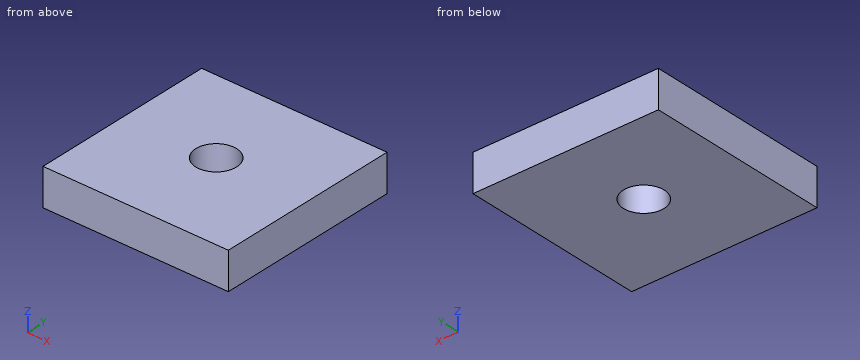
from build123d import *

# Parameters (mm, degrees)
F1_W     = 12.7
F1_H     = 12.7
F2_DEPTH = 2.54
F0_R     = 1.397
F3_DEPTH = 22.7076


with BuildPart() as f2:
    # F1 (on Top) → F2 (new body)
    with BuildSketch(Plane.XY):
        with Locations((0.047929, -0.151867)):
            Rectangle(F1_W, F1_H)
    extrude(amount=F2_DEPTH)

    # F0 (on Top) → F3 (cut)
    with BuildSketch(Plane.XY):
        Circle(F0_R)
    extrude(amount=F3_DEPTH, mode=Mode.SUBTRACT)


solid = f2.part
For this review, take the finished solid that the model builds, in its own axes (mm). Round coordinates to 2 decimals unless told otherwise and drop trailing zeros. Order: outer loops, then holes, each group sorted by start corner. A loop starts at its lowest first (then second) coordinate and runs counter-clockwise, first axis right, second up. Notation, with made-up numbers: M -33.5,-28.75 L -12.5,-28.75 A15 ccw -12.5,-11.75 Z; hole C 64.25,-18 d4. An arc over 180 degrees is marked long. Use a Markdown table: item, result. Add a question column.
Item 1: Add section C-C, the plane z = 2.2. Give the boundary of the cut face in (x, y).
Item 2: Add section B-B, the plane y = 0. Give the boundary of the cut face in (x, z), then the cut area to 3 significant figures.
Item 3: Insertion check: pin 1 (2 mm diameter, centred on x = 0, y = 0, fed in from -Z). The pin has a flat end and moves straight along its axis. Give the tip position at first contact, or say it passes through.
Item 4: Add section A-A, the plane x = 0. Give the boundary of the cut face in (y, z), then the cut area to 3 significant figures.
Item 5: To check wall thickness, follow line 1 along Y through (x, z) = (0, 0.6); line 2 along X through (y, z) = (0, 1.45); line 3 along Y through (x, z) = (1, 2.45). State the ranges of each line that lie inside material, in increasing order.
Geometry results:
| question | item | result |
|---|---|---|
| 1 | outline | M -6.3,-6.5 L 6.4,-6.5 L 6.4,6.2 L -6.3,6.2 Z; hole C 0,0 d2.79 |
| 2 | outline | M -6.3,0 L -1.4,0 L -1.4,2.54 L -6.3,2.54 Z; M 1.4,0 L 6.4,0 L 6.4,2.54 L 1.4,2.54 Z |
| 2 | area | 25.2 mm² |
| 3 | pin 1 | passes through |
| 4 | outline | M -6.5,0 L -1.4,0 L -1.4,2.54 L -6.5,2.54 Z; M 1.4,0 L 6.2,0 L 6.2,2.54 L 1.4,2.54 Z |
| 4 | area | 25.2 mm² |
| 5 | line 1 | y = -6.5 to -1.4, 1.4 to 6.2 |
| 5 | line 2 | x = -6.3 to -1.4, 1.4 to 6.4 |
| 5 | line 3 | y = -6.5 to -0.98, 0.98 to 6.2 |
